The model under review builds one solid part; all positions refer to its coordinate system, in mm. Face numbers are marked on the shaded views. Round coordinates to 2 decimals unless told otherwise and drop trailing zeros. Write each loop counter-clockwise with the first axis right and the second up, starting at its lowest first coordinate (ties: lowest second). Pieces come first, ordered by that corner, then holes. Notation, with made-up numbers: M 89.25,64.25 L 130.25,64.25 A22 cw 130.25,70.25 Z; hole C -37,86 d8. An arc over 180 degrees is marked long. Write item = value, one per line. Start each with the question number.
Item 1: Take a section at A-A, the plane x = 18.5. Give the boundary of the cut face in (y, z).
Item 2: Take a section at C-C, the plane x = -24. Give the boundary of the cut face in (y, z).
Item 3: For pin 1 Ø0.6 at (x, z) = (16.87, -20.05) entering from -Y; pin 2 Ø0.9 at (x, y) = (40, 1) entering from +Z; pin 3 Ø1 at (y, z) = (2, -7.5) entering from -X; pin 4 Ø1 at (x, y) = (-21.5, 1) entering from +Z, all flat-tipped, find the tip position at first contact; note any pin that passes through.
Item 4: Take a section at B-B, the plane z = -12. Give the boundary of the cut face in (x, y).
Item 5: To check wall thickness, follow line 1 along X through (y, z) = (1.4, -9.25); line 2 along X through (y, z) = (2.1, -11); line 3 along X through (y, z) = (1.7, -16). State the ranges of each line that lie inside material, in increasing order.
Item 6: The part is to be moulded in two halves that separate along Y. For the marked faces 1 and 2, say which applies: +Y half, -Y half, draft (parallel to the pull), parting line (faces both ways), or undercut.
Item 7: Take a section at D-D, the plane y = 1.7. Give the number of separate pieces and of enclosed holes in the cut face, plus the area to 3 significant figures.
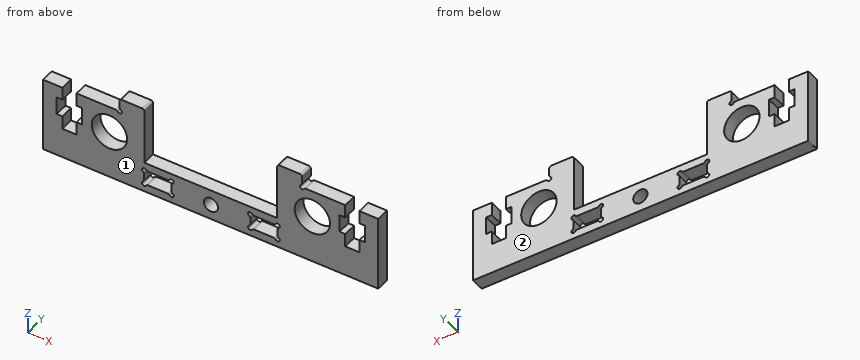
from build123d import *

# Parameters (mm, degrees)
SKETCH1_R           = 4.009255558
SKETCH1_R_2         = 1.619702369
BOSS_EXTRUDE1_DEPTH = 3


with BuildPart() as part:
    # Sketch1 → Boss-Extrude1 (new body)
    with BuildSketch(Plane(origin=(0, 0, 0), x_dir=(1, 0, 0), z_dir=(0, 1, 0))):
        with BuildLine():
            Line((-7.143850408, 18.229298667), (22.987065755, 18.229298667))
            Line((22.987065755, 18.229298667), (22.987065755, 7.324979297))
            Line((22.987065755, 7.324979297), (22.987065755, 5.690951323))
            ThreePointArc((22.987065755, 5.690951323), (23.133512364, 5.337397932), (23.487065755, 5.190951323))
            Line((23.487065755, 5.190951323), (28.129403654, 5.190951323))
            ThreePointArc((28.129403654, 5.190951323), (28.482956988, 5.337397909), (28.629403574, 5.690951243))
            Line((28.629403574, 5.690951243), (28.629403574, 7.324979243))
            ThreePointArc((28.629403574, 7.324979243), (28.56241665, 7.574978633), (28.379404865, 7.757991282))
            ThreePointArc((28.379404865, 7.757991282), (28.275853546, 8.544556775), (29.062418723, 8.441003056))
            ThreePointArc((29.062418723, 8.441003056), (29.245431425, 8.257990354), (29.495431425, 8.191003056))
            Line((29.495431425, 8.191003056), (38.401967533, 8.191003056))
            Line((38.401967533, 8.191003056), (38.401967533, 11.193716571))
            Line((38.401967533, 11.193716571), (37.120165143, 11.193716571))
            Line((37.120165143, 11.193716571), (37.120165143, 15.215104531))
            Line((37.120165143, 15.215104531), (38.40196755, 15.215104531))
            Line((38.40196755, 15.215104531), (38.40196755, 18.231124388))
            Line((38.40196755, 18.231124388), (41.619067462, 18.231124388))
            Line((41.619067462, 18.231124388), (41.619067462, 15.215104531))
            Line((41.619067462, 15.215104531), (42.900869869, 15.215104531))
            Line((42.900869869, 15.215104531), (42.900869869, 11.193716571))
            Line((42.900869869, 11.193716571), (41.619067445, 11.193716571))
            Line((41.619067445, 11.193716571), (41.619067445, 8.191003056))
            Line((41.619067445, 8.191003056), (45.879856116, 8.191003056))
            Line((45.879856116, 8.191003056), (45.879856116, 25.171092004))
            Line((45.879856116, 25.171092004), (-29.989227631, 25.171092004))
            ThreePointArc((-29.989227631, 25.171092004), (-30.077254418, 25.14100432), (-30.109006218, 25.053564013))
            Line((-30.109006218, 25.053564013), (-30.109006218, 8.29196371))
            Line((-30.109006218, 8.29196371), (-25.72867026, 8.29196371))
            Line((-25.72867026, 8.29196371), (-25.72867026, 11.238755399))
            Line((-25.72867026, 11.238755399), (-27.010472684, 11.238755399))
            Line((-27.010472684, 11.238755399), (-27.010472684, 15.260143358))
            Line((-27.010472684, 15.260143358), (-25.728670277, 15.260143358))
            Line((-25.728670277, 15.260143358), (-25.728670277, 18.276163216))
            Line((-25.728670277, 18.276163216), (-22.511570365, 18.276163216))
            Line((-22.511570365, 18.276163216), (-22.511570365, 15.260143358))
            Line((-22.511570365, 15.260143358), (-21.229767957, 15.260143358))
            Line((-21.229767957, 15.260143358), (-21.229767957, 11.238755399))
            Line((-21.229767957, 11.238755399), (-22.511570348, 11.238755399))
            Line((-22.511570348, 11.238755399), (-22.511570348, 8.236041884))
            Line((-22.511570348, 8.236041884), (-13.60503424, 8.236041884))
            ThreePointArc((-13.60503424, 8.236041884), (-13.356468602, 8.303656274), (-13.174549931, 8.486035491))
            ThreePointArc((-13.174549931, 8.486035491), (-12.387984754, 8.58958921), (-12.491536073, 7.803023717))
            ThreePointArc((-12.491536073, 7.803023717), (-12.674547858, 7.620011069), (-12.741534782, 7.370011678))
            Line((-12.741534782, 7.370011678), (-12.741534782, 5.735983678))
            ThreePointArc((-12.741534782, 5.735983678), (-12.595088173, 5.382430288), (-12.241534782, 5.235983678))
            Line((-12.241534782, 5.235983678), (-7.653939136, 5.235983678))
            ThreePointArc((-7.653939136, 5.235983678), (-7.309014548, 5.362697937), (-7.143850408, 5.690951317))
            Line((-7.143850408, 5.690951317), (-7.143850408, 7.324979297))
            Line((-7.143850408, 7.324979297), (-7.143850408, 18.229298667))
        make_face()
        with Locations((-15.055624081, 14.270241393)):
            Circle(SKETCH1_R, mode=Mode.SUBTRACT)
        with Locations((30.946299637, 14.270241393)):
            Circle(SKETCH1_R, mode=Mode.SUBTRACT)
        with BuildLine():
            ThreePointArc((-6.750210098, 23.598159475), (-6.567197449, 23.415147689), (-6.317198059, 23.348160765))
            Line((-6.317198059, 23.348160765), (-1.849249059, 23.348160765))
            ThreePointArc((-1.849249059, 23.348160765), (-1.599248991, 23.415148256), (-1.41623632, 23.598161152))
            ThreePointArc((-1.41623632, 23.598161152), (-0.629670838, 23.701715154), (-0.733222121, 22.915149315))
            ThreePointArc((-0.733222121, 22.915149315), (-0.916234557, 22.73213507), (-0.983220424, 22.482133752))
            Line((-0.983220424, 22.482133752), (-0.983220424, 20.914266752))
            ThreePointArc((-0.983220424, 20.914266752), (-0.916233017, 20.664266494), (-0.733220037, 20.481253678))
            ThreePointArc((-0.733220037, 20.481253678), (-0.629666036, 19.694688196), (-1.416231875, 19.798239479))
            ThreePointArc((-1.416231875, 19.798239479), (-1.599244524, 19.981251265), (-1.849243914, 20.048238189))
            Line((-1.849243914, 20.048238189), (-6.317193914, 20.048238189))
            ThreePointArc((-6.317193914, 20.048238189), (-6.567193914, 19.981250891), (-6.750206616, 19.798238189))
            ThreePointArc((-6.750206616, 19.798238189), (-7.536772071, 19.694684496), (-7.433220534, 20.481250235))
            ThreePointArc((-7.433220534, 20.481250235), (-7.250208657, 20.664263235), (-7.18322203, 20.91426303))
            Line((-7.18322203, 20.91426303), (-7.18322203, 22.48213303))
            ThreePointArc((-7.18322203, 22.48213303), (-7.250209567, 22.732132487), (-7.43322203, 22.915144775))
            ThreePointArc((-7.43322203, 22.915144775), (-7.536776448, 23.701710706), (-6.750210098, 23.598159475))
        make_face(mode=Mode.SUBTRACT)
        with Locations((7.945337781, 21.71531407)):
            Circle(SKETCH1_R_2, mode=Mode.SUBTRACT)
        with BuildLine():
            Line((17.739921148, 23.348159476), (22.207870148, 23.348159476))
            ThreePointArc((22.207870148, 23.348159476), (22.457869729, 23.415146316), (22.640882523, 23.598158186))
            ThreePointArc((22.640882523, 23.598158186), (23.427448874, 23.701709417), (23.323894455, 22.915143486))
            ThreePointArc((23.323894455, 22.915143486), (23.140882484, 22.732132355), (23.073894191, 22.482134307))
            Line((23.073894191, 22.482134307), (23.073894191, 20.914264307))
            ThreePointArc((23.073894191, 20.914264307), (23.140881057, 20.664265055), (23.323892694, 20.481252469))
            ThreePointArc((23.323892694, 20.481252469), (23.427444232, 19.69468673), (22.640878777, 19.798240423))
            ThreePointArc((22.640878777, 19.798240423), (22.457866075, 19.981253125), (22.207866075, 20.048240423))
            Line((22.207866075, 20.048240423), (17.739916075, 20.048240423))
            ThreePointArc((17.739916075, 20.048240423), (17.489916684, 19.981253499), (17.306904036, 19.798241714))
            ThreePointArc((17.306904036, 19.798241714), (16.520338196, 19.69469043), (16.623892198, 20.481255912))
            ThreePointArc((16.623892198, 20.481255912), (16.806904939, 20.664268314), (16.873892585, 20.91426803))
            Line((16.873892585, 20.91426803), (16.873892585, 22.48213503))
            ThreePointArc((16.873892585, 22.48213503), (16.8069059, 22.732134962), (16.623893876, 22.915148025))
            ThreePointArc((16.623893876, 22.915148025), (16.520342592, 23.701713865), (17.306908074, 23.598159863))
            ThreePointArc((17.306908074, 23.598159863), (17.48992089, 23.415146883), (17.739921148, 23.348159476))
        make_face(mode=Mode.SUBTRACT)
    extrude(amount=BOSS_EXTRUDE1_DEPTH)


solid = part.part
Response values:
q1.outline = M 0,-25.17 L 3,-25.17 L 3,-23.35 L 0,-23.35 Z; M 0,-20.05 L 3,-20.05 L 3,-18.23 L 0,-18.23 Z
q2.outline = M 0,-25.17 L 3,-25.17 L 3,-18.28 L 0,-18.28 Z
q3.pin_1 = through
q3.pin_2 = -18.23
q3.pin_3 = -12.74
q3.pin_4 = -8.24
q4.outline = M -30.11,0 L -27.01,0 L -27.01,3 L -30.11,3 Z; M -21.23,0 L -18.36,0 L -18.36,3 L -21.23,3 Z; M -11.75,0 L -7.14,0 L -7.14,3 L -11.75,3 Z; M 22.99,0 L 27.64,0 L 27.64,3 L 22.99,3 Z; M 34.25,0 L 37.12,0 L 37.12,3 L 34.25,3 Z; M 42.9,0 L 45.88,0 L 45.88,3 L 42.9,3 Z
q5.line_1 = -30.11 to -25.73, -22.51 to -7.14, 22.99 to 38.4, 41.62 to 45.88
q5.line_2 = -30.11 to -25.73, -22.51 to -17.38, -12.74 to -7.14, 22.99 to 28.63, 33.27 to 38.4, 41.62 to 45.88
q5.line_3 = -30.11 to -25.73, -22.51 to -18.67, -11.44 to -7.14, 22.99 to 27.33, 34.56 to 38.4, 41.62 to 45.88
q6.face_1 = -Y half
q6.face_2 = +Y half
q7.separate_pieces = 1
q7.enclosed_holes = 5
q7.area = 778 mm2
